Check sheet for the modelled part. Datum: model origin and axes. Units: mm. A direction names the side the tool comes from. Round coordinates to 2 decimals unless told otherwise and drop trailing zeros. Write each loop counter-clockwise with the first axis right and the second up, starting at its lowest first coordinate (ties: lowest second). Pieces come first, ordered by that corner, then holes. Notation, with made-up numbers: (50.25, -36) -> (99.25, -36) arc R3 ccw to (99.25, -32) -> close; hole circle Ø8 at (-39, 50). An arc over 180 degrees is marked (long way). One line per item, written item: value.
Autodesk Inventor part; units mm, degrees
ref_plane "YZ Plane" through (0, 0, 0) normal (1, 0, 0) x (0, 1, 0)
ref_plane "XZ Plane" through (0, 0, 0) normal (0, 1, 0) x (-1, 0, 0)
ref_plane "XY Plane" through (0, 0, 0) normal (0, 0, 1) x (1, 0, 0)
sketch "Эскиз1" plane through (0, 0, 0) normal (0, 0, 1) x (1, 0, 0)
  line L0 (83.9845, -81.4877) -> (83.9845, -84.9877)
  line L1 (47.9845, -84.9877) -> (47.9845, -81.4877)
  line L2 (64.2345, -65.2377) -> (67.7345, -65.2377)
  line L3 (67.7345, -101.2377) -> (64.2345, -101.2377)
  circle A0 centre (49.7345, -83.2377) radius 0.75
  circle A1 centre (52.7345, -83.2377) radius 0.75
  circle A2 centre (55.7345, -83.2377) radius 0.75
  circle A3 centre (58.7345, -83.2377) radius 0.75
  circle A4 centre (82.2345, -83.2377) radius 0.75
  circle A5 centre (79.2345, -83.2377) radius 0.75
  circle A6 centre (76.2345, -83.2377) radius 0.75
  circle A7 centre (73.2345, -83.2377) radius 0.75
  circle A8 centre (65.9845, -99.4877) radius 0.75
  circle A9 centre (65.9845, -96.4877) radius 0.75
  circle A10 centre (65.9845, -93.4877) radius 0.75
  circle A11 centre (65.9845, -90.4877) radius 0.75
  circle A12 centre (65.9845, -66.9877) radius 0.75
  circle A13 centre (65.9845, -69.9877) radius 0.75
  circle A14 centre (65.9845, -72.9877) radius 0.75
  circle A15 centre (65.9845, -75.9877) radius 0.75
  line L4 (49.9845, -79.4877) -> (60.2345, -79.4877)
  line L5 (71.7345, -79.4877) -> (81.9845, -79.4877)
  line L6 (62.2345, -99.2377) -> (62.2345, -88.9877)
  line L7 (62.2345, -77.4877) -> (62.2345, -67.2377)
  line L8 (81.9845, -86.9877) -> (71.7345, -86.9877)
  line L9 (60.2345, -86.9877) -> (49.9845, -86.9877)
  line L10 (69.7345, -67.2377) -> (69.7345, -77.4877)
  line L11 (69.7345, -88.9877) -> (69.7345, -99.2377)
  circle A16 centre (65.9845, -83.2377) radius 4.25
  circle A17 centre (65.9845, -83.2377) radius 2.75
  arc A18 (60.2345, -79.4877) -> (62.2345, -77.4877) centre (60.2345, -77.4877) ccw
  arc A19 (62.2345, -88.9877) -> (60.2345, -86.9877) centre (60.2345, -88.9877) ccw
  arc A20 (71.7345, -86.9877) -> (69.7345, -88.9877) centre (71.7345, -88.9877) ccw
  arc A21 (69.7345, -77.4877) -> (71.7345, -79.4877) centre (71.7345, -77.4877) ccw
  arc A22 (83.9845, -81.4877) -> (81.9845, -79.4877) centre (81.9845, -81.4877) ccw
  arc A23 (81.9845, -86.9877) -> (83.9845, -84.9877) centre (81.9845, -84.9877) ccw
  arc A24 (69.7345, -67.2377) -> (67.7345, -65.2377) centre (67.7345, -67.2377) ccw
  arc A25 (64.2345, -65.2377) -> (62.2345, -67.2377) centre (64.2345, -67.2377) ccw
  arc A26 (49.9845, -79.4877) -> (47.9845, -81.4877) centre (49.9845, -81.4877) ccw
  arc A27 (47.9845, -84.9877) -> (49.9845, -86.9877) centre (49.9845, -84.9877) ccw
  arc A28 (62.2345, -99.2377) -> (64.2345, -101.2377) centre (64.2345, -99.2377) ccw
  arc A29 (67.7345, -101.2377) -> (69.7345, -99.2377) centre (67.7345, -99.2377) ccw
  circle A30 centre (65.9845, -83.2377) radius 1.5
  point P0 (0, 0)
  point P1 (83.9845, -79.4877)
  point P2 (83.9845, -86.9877)
  point P3 (62.2345, -65.2377)
  point P4 (69.7345, -65.2377)
  point P5 (69.7345, -101.2377)
  point P6 (62.2345, -101.2377)
  dimension "d4" = 7.5
  dimension "d6" = 7.5
  dimension "d7" = 7.5
  dimension "d9" = 1.5
  dimension "d11" = 1.5
  dimension "d13" = 1.5
  dimension "d15" = 1.5
  dimension "d17" = 1.5
  dimension "d19" = 1.5
  dimension "d21" = 1.5
  dimension "d23" = 1.5
  dimension "d24" = 8.5
  dimension "d25" = 5.5
  dimension "d26" = 2
  dimension "d27" = 3
extrude "Выдавливание1" add sketch "Эскиз1" along normal blind 2 contours L0 A23 L8 A20 L11 A29 L3 A28 L6 A19 L9 A27 L1 A26 L4 A18 L7 A25 L2 A24 L10 A21 L5 A22
extrude "Выдавливание2" add sketch "Эскиз1" along normal blind 5 contours A16
extrude "Выдавливание3" add sketch "Эскиз1" along normal blind 2 contours A17
properties part number "Звезда"
Item 1: Sectioned sample at D-D on z = 0.65. Count the separate pieces of the cut face and the enclosed holes in it, and give its area (3 significant figures).
Answer:
separate pieces: 1
enclosed holes: 17
area: 445 mm^2
Item 2: Depth check by flat-ended pin: P1, Ø2, axis at y = -73.5, z = 0.5, coming from the +X side; P2, Ø1.4, axis at x = 65.98, y = -72.99, coming from the +Z side; P3, Ø3, axis at x = 69.5, y = -93.5, coming from the -Z side; P4, Ø2, axis at y = -94.5, z = 0.5, coming from the -X side. Enter the tip coordinate at first touch or a pass-through.
Answer:
P1: stops at x = 69.73
P2: passes through
P3: stops at z = 0
P4: stops at x = 62.23
Item 3: Sectioned sample at C-C on z = 4.2. Enter the section's corners in (x, y), and give its area (3 significant figures).
Answer:
outline: circle Ø8.5 at (65.98, -83.24); hole circle Ø5.5 at (65.98, -83.24)
area: 33.0 mm^2
Item 4: Sectioned sample at B-B on y = -80. Enter the section's corners in (x, z).
Answer:
outline: (48.65, 0) -> (83.32, 0) -> (83.32, 2) -> (68.74, 2) -> (68.74, 5) -> (63.23, 5) -> (63.23, 2) -> (48.65, 2) -> close
Item 5: Mould release check, pull along Y, two halves, no side actions. Record for faces 5 (the flat face through (55, -86.988, 1)), 6 (the flat face through (62.234, -94, 1)), 7 (the cylindrical face through (72.64, -82.78, 0.99)): pulls with the +Y half, pulls with the -Y half, needs draft (parallel to the pull), parting line crosses it, or undercut.
Answer:
face 5: pulls with the -Y half
face 6: needs draft
face 7: undercut
Item 6: Tool access check on faces 1 (the flat face through (62.234, -72, 1)), 2 (the flat face through (62, -80, 2)), 3 (the flat face through (77, -86.988, 1)), 4 (the flat face through (69.734, -72, 1)). Record the directions out of +Z, -Z, +X, -X, +Y, -Y that give a thin tool (end or side, any length) a straight path to the whole face; none if there is none.
Answer:
face 1: +Z, -Z, -X, +Y
face 2: +Z
face 3: +Z, -Z, +X, -Y
face 4: +Z, -Z, +X, +Y
Item 7: Sectioned sample at A-A on x = 76. Enter the section's corners in (y, z).
Answer:
outline: (-86.99, 0) -> (-83.95, 0) -> (-83.95, 2) -> (-86.99, 2) -> close; (-82.53, 0) -> (-79.49, 0) -> (-79.49, 2) -> (-82.53, 2) -> close
Item 8: Thickness scan on line 1 (X direction, y = -96.5, z = 1.15); line 2 (Z direction, x = 51.5, y = -80); line 3 (Y direction, x = 79.5, z = 1.3). Record the ranges inside material, lowest first.
Answer:
line 1: x = 62.23 to 65.23, 66.73 to 69.73
line 2: z = 0 to 2
line 3: y = -86.99 to -83.94, -82.54 to -79.49
